```python
from build123d import *

# Parameters (mm, degrees)
F0_W     = 100
F0_H     = 100
F1_DEPTH = 50
F2_R     = 17.5
F3_DEPTH = 100
F4_R     = 17.5
F5_DEPTH = 100
F6_R     = 17.5
F7_DEPTH = 100
F8_R     = 10


with BuildPart() as f1:
    # F0 (on Front) → F1 (new body, symmetric)
    with BuildSketch(Plane.XZ):
        Rectangle(F0_W, F0_H)
    extrude(amount=F1_DEPTH, both=True)

    # F2 (on face) → F3 (cut, through all)
    with BuildSketch(Plane.XZ.offset(50)):
        Circle(F2_R)
    extrude(amount=-F3_DEPTH, mode=Mode.SUBTRACT)

    # F4 (on face) → F5 (cut, through all)
    with BuildSketch(Plane.YZ.offset(50)):
        Circle(F4_R)
    extrude(amount=-F5_DEPTH, mode=Mode.SUBTRACT)

    # F6 (on face) → F7 (cut, through all)
    with BuildSketch(Plane.XY.offset(50)):
        Circle(F6_R)
    extrude(amount=-F7_DEPTH, mode=Mode.SUBTRACT)

    # F8
    f8_edges = [f1.edges().sort_by_distance(p)[0] for p in [
        (50, 0, 50),
        (50, 50, 0),
        (50, 0, -50),
        (50, -50, 0),
        (0, -50, 50),
        (-50, 0, 50),
        (0, 50, 50),
        (-50, 50, 0),
        (0, 50, -50),
        (-50, 0, -50),
        (-50, -50, 0),
        (0, -50, -50),
    ]]
    fillet(f8_edges, radius=F8_R)


solid = f1.part
```
Read the model definition and answer for the solid it produces. Units are mm, in the model's axes. Give positions to 0.01 mm unless a question says otherwise; leave off trailing zeros. Order: outer loops, then holes, each group sorted by start corner. A loop starts at its lowest first (then second) coordinate and runs counter-clockwise, first axis right, second up.
(1) A straight line is drawn through the part: L1, parallel to X at y = 33, z = 0. Find the intervals that lie inside material, in ascending order.
(2) For a pull along X with two mould halves and no side action, classify faces 1 (the cylindrical face through (-17.483, 0.769, -30.924)), 2 (the flat face through (50, -18, -1)), 3 (the cylindrical face through (31.451, -17.483, 0.769)) as released by +X, released by -X, zero draft, split by the parting line, or undercut.
(3) Find section C-C (y = -34). Give the vertices of the cut face in (x, z), plus the area to 3 significant figures.
(4) Given pin 1 (5 mm diameter, centred on x = 13, y = 8, fed in from -Z), flat-ended and moving along its own axis, determine where the tip first touches the part or whether it passes through.
(5) Find section A-A (z = 0). Give the vertices of the cut face in (x, y), plus the area to 3 significant figures.
Result sheet:
1. L1: x = -50 to -17.5, 17.5 to 50
2. face 1: undercut
2. face 2: released by +X
2. face 3: zero draft
3. outline: (-50, -40) arc R10 ccw to (-40, -50) - (40, -50) arc R10 ccw to (50, -40) - (50, 40) arc R10 ccw to (40, 50) - (-40, 50) arc R10 ccw to (-50, 40) - close; hole circle Ø35 at (0, 0)
3. area: 8,950 mm2
4. pin 1: stops at z = -50
5. outline: (-50, -40) arc R10 ccw to (-40, -50) - (-17.5, -50) - (-17.5, -17.5) - (-50, -17.5) - close; (-50, 17.5) - (-17.5, 17.5) - (-17.5, 50) - (-40, 50) arc R10 ccw to (-50, 40) - close; (17.5, -50) - (40, -50) arc R10 ccw to (50, -40) - (50, -17.5) - (17.5, -17.5) - close; (17.5, 17.5) - (50, 17.5) - (50, 40) arc R10 ccw to (40, 50) - (17.5, 50) - close
5. area: 4,140 mm2
